```python
from build123d import *

# Parameters (mm, degrees)
ESQUISSE4_R        = 10
ESQUISSE4_R_2      = 15
BOSS_EXTRU_1_DEPTH = 3
D_GAGEMENT_M51_D   = 5.5


with BuildPart() as part:
    # Esquisse4 → Boss.-Extru.1 (new body)
    with BuildSketch(Plane.XY):
        with Locations((145.009245926, 102.618921879)):
            Circle(ESQUISSE4_R)
        with BuildLine():
            Line((36.96319164, 36.860248406), (149.516585657, 93.692338627))
            ThreePointArc((149.516585657, 93.692338627), (135.946168055, 98.392739261), (141.068348562, 111.809641544))
            Line((141.068348562, 111.809641544), (-5.911346046, 48.786079498))
            ThreePointArc((-5.911346046, 48.786079498), (8.25620401, 47.523381945), (15, 35))
            ThreePointArc((15, 35), (14.961488006, 33.925813491), (14.846149779, 32.857142857))
            Line((14.846149779, 32.857142857), (13.730743914, 25.129384342))
            Line((13.730743914, 25.129384342), (36.96319164, 36.860248406))
        make_face()
        with Locations((0, 35)):
            Circle(ESQUISSE4_R_2)
        with BuildLine():
            Line((10.012724365, -0.629810709), (13.730743914, 25.129384342))
            Line((13.730743914, 25.129384342), (6.761009597, 21.610125123))
            ThreePointArc((6.761009597, 21.610125123), (-6.925765295, 21.69459602), (-14.846149779, 32.857142857))
            Line((-14.846149779, 32.857142857), (-9.897433186, -1.428571429))
            ThreePointArc((-9.897433186, -1.428571429), (-0.716124339, 9.974325337), (10, 0))
            ThreePointArc((10, 0), (9.974325337, -0.716124339), (9.897433186, -1.428571429))
            Line((9.897433186, -1.428571429), (10.012724365, -0.629810709))
        make_face()
        Circle(ESQUISSE4_R)
        with BuildLine():
            ThreePointArc((10.012724365, -0.629810709), (18.9014248, 21.412338562), (36.96319164, 36.860248406))
            Line((36.96319164, 36.860248406), (13.730743914, 25.129384342))
            Line((13.730743914, 25.129384342), (10.012724365, -0.629810709))
        make_face()
        with BuildLine():
            Line((6.761009597, 21.610125123), (13.730743914, 25.129384342))
            Line((13.730743914, 25.129384342), (14.846149779, 32.857142857))
            ThreePointArc((14.846149779, 32.857142857), (12.179539649, 26.244498076), (6.761009597, 21.610125123))
        make_face()
    extrude(amount=BOSS_EXTRU_1_DEPTH)

    # Dégagement M51 (through all)
    with Locations(Plane(origin=(0, 0, 3), x_dir=(-1, 0, 0), z_dir=(0, 0, 1))):
        with Locations((-145.009245926, -102.618921879), (0, -35), (0, 0)):
            Hole(D_GAGEMENT_M51_D / 2)


solid = part.part
```
Work out the finished part from the listing and answer in its coordinate system (mm). Give positions to 0.01 mm unless a question says otherwise; leave off trailing zeros. Loops run counter-clockwise (first coordinate to the right, second up) from the corner with the lowest first, then second, coordinate; pieces in that order, holes last. Notation, with made-up numbers: (-7.75, 2.5) -> (0.25, 2.5) arc R33 cw to (0.25, 40.5) -> close; hole circle Ø11 at (89, 7.5). An arc over 180 degrees is marked (long way). Put each result on its own line as item: value. Start each with the question number.
Item 1: The part is cut by section B-B (y = 35). Give the vertices of the cut face in (x, z).
Item 2: Each of these flat-tipped pins is pushed along its axis until it touches: P1, Ø6.5, axis at x = 0, y = 0, coming from the +Z side; P2, Ø4.5, axis at x = 0, y = 35, coming from the -Z side; P3, Ø1.5, axis at y = 79, z = 2.5, coming from the +X side. Where does it stop, or does it pass through?
Item 3: The part is cut by section A-A (x = 0). Give the vertices of the cut face in (y, z).
Item 4: The part is cut by section D-D (x = 115.5). Give the vertices of the cut face in (y, z).
Item 5: The part is cut by section C-C (z = 2.25). Give the vertices of the cut face in (x, y).
Item 6: The mould has two halves that part along Y. Classify faces 1 (the face through (57, 61, 3)), 2 (the face through (-0.358, 32.273, 1.479)), 3 (the face through (147.63, 101.79, 1.48)), 4 (the face through (154, 107, 1)): released by +Y, released by -Y, zero draft, split by the parting line, or undercut.
Item 7: Find the intervals of material crossed by L1, parallel to Y at x = 0, z = 2.05; L2, parallel to X at y = 34, z = 2.7; L3, parallel to X at y = 104, z = 0.5, in increasing order. Write a range as [from, to].
Answers below:
1. outline: (-15, 0) -> (-2.75, 0) -> (-2.75, 3) -> (-15, 3) -> close; (2.75, 0) -> (33.61, 0) -> (33.61, 3) -> (2.75, 3) -> close
2. P1: z = 3
2. P2: through
2. P3: x = 121.9
3. outline: (-10, 0) -> (-2.75, 0) -> (-2.75, 3) -> (-10, 3) -> close; (2.75, 0) -> (32.25, 0) -> (32.25, 3) -> (2.75, 3) -> close; (37.75, 0) -> (51.32, 0) -> (51.32, 3) -> (37.75, 3) -> close
4. outline: (76.52, 0) -> (100.85, 0) -> (100.85, 3) -> (76.52, 3) -> close
5. outline: (-14.85, 32.86) -> (-9.9, -1.43) arc R10 ccw to (9.9, -1.43) -> (10.01, -0.63) arc R50 cw to (36.96, 36.86) -> (149.52, 93.69) arc R10 ccw to (141.07, 111.81) -> (-5.91, 48.79) arc R15 ccw to start; hole circle Ø5.5 at (0, 0); hole circle Ø5.5 at (0, 35); hole circle Ø5.5 at (145.01, 102.62)
6. face 1: zero draft
6. face 2: undercut
6. face 3: undercut
6. face 4: split by the parting line
7. L1: [-10, -2.75], [2.75, 32.25], [37.75, 51.32]
7. L2: [-14.97, -2.56], [2.56, 32.02]
7. L3: [122.86, 142.63], [147.39, 154.91]
